```python
from build123d import *

# Parameters (mm, degrees)
PARED_DEPTH           = 25
CONECTORES_REACH      = 165.441
CROQUIS2_W            = 15
CROQUIS2_H            = 13
CROQUIS2_W_2          = 12
CROQUIS2_H_2          = 7
BASE_START            = -1.12
BASE_FRENTE_DEPTH     = 1.12
CORTAR_EXTRUIR2_REACH = 164.686
CROQUIS3_W            = 2
CROQUIS3_H            = 5.5


with BuildPart() as part:
    # Croquis1 → pared (new body)
    with BuildSketch(Plane.XY):
        with BuildLine():
            Line((9, 76.1), (131, 76.1))
            ThreePointArc((131, 76.1), (138.495331881, 72.995331881), (141.6, 65.5))
            Line((141.6, 65.5), (141.6, 9))
            ThreePointArc((141.6, 9), (138.495331881, 1.504668119), (131, -1.6))
            Line((131, -1.6), (9, -1.6))
            ThreePointArc((9, -1.6), (1.504668119, 1.504668119), (-1.6, 9))
            Line((-1.6, 9), (-1.6, 65.5))
            ThreePointArc((-1.6, 65.5), (1.504668119, 72.995331881), (9, 76.1))
        make_face()
        with BuildLine():
            Line((9, 0), (131, 0))
            ThreePointArc((131, 0), (137.363961031, 2.636038969), (140, 9))
            Line((140, 9), (140, 65.5))
            ThreePointArc((140, 65.5), (137.363961031, 71.863961031), (131, 74.5))
            Line((131, 74.5), (9, 74.5))
            ThreePointArc((9, 74.5), (2.636038969, 71.863961031), (0, 65.5))
            Line((0, 65.5), (0, 9))
            ThreePointArc((0, 9), (2.636038969, 2.636038969), (9, 0))
        make_face(mode=Mode.SUBTRACT)
    extrude(amount=PARED_DEPTH)

    # Croquis2 → conectores (cut, up to next)
    with BuildSketch(Plane.XZ.offset(1.6), mode=Mode.PRIVATE) as conectores_sk1:
        with Locations((111, 9.5)):
            Rectangle(CROQUIS2_W, CROQUIS2_H)
    conectores_tool1 = extrude(conectores_sk1.sketch, amount=-CONECTORES_REACH, mode=Mode.PRIVATE) & part.part
    # Croquis2 → conectores (cut, up to next)
    with BuildSketch(Plane.XZ.offset(1.6), mode=Mode.PRIVATE) as conectores_sk2:
        with Locations((96, 14.5)):
            Rectangle(CROQUIS2_W_2, CROQUIS2_H_2)
    conectores_tool2 = extrude(conectores_sk2.sketch, amount=-CONECTORES_REACH, mode=Mode.PRIVATE) & part.part
    add(conectores_tool1.solids().sort_by_distance((111, -1.6, 9.5))[0], mode=Mode.SUBTRACT)
    add(conectores_tool2.solids().sort_by_distance((96, -1.6, 14.5))[0], mode=Mode.SUBTRACT)

    # Croquis1_2 → base frente (add)
    with BuildSketch(Plane.XY.offset(BASE_START)):
        with BuildLine():
            Line((9, 76.1), (131, 76.1))
            ThreePointArc((131, 76.1), (138.495331881, 72.995331881), (141.6, 65.5))
            Line((141.6, 65.5), (141.6, 9))
            ThreePointArc((141.6, 9), (138.495331881, 1.504668119), (131, -1.6))
            Line((131, -1.6), (9, -1.6))
            ThreePointArc((9, -1.6), (1.504668119, 1.504668119), (-1.6, 9))
            Line((-1.6, 9), (-1.6, 65.5))
            ThreePointArc((-1.6, 65.5), (1.504668119, 72.995331881), (9, 76.1))
        make_face()
    extrude(amount=BASE_FRENTE_DEPTH)

    # Croquis3 → Cortar-Extruir2 (cut, up to next)
    with BuildSketch(Plane.XY, mode=Mode.PRIVATE) as cortar_extruir2_sk1:
        with BuildLine():
            Line((131.5, 13), (132.5, 13))
            ThreePointArc((132.5, 13), (132.853553391, 13.146446609), (133, 13.5))
            Line((133, 13.5), (133, 27.5))
            ThreePointArc((133, 27.5), (132.853553391, 27.853553391), (132.5, 28))
            Line((132.5, 28), (131.5, 28))
            ThreePointArc((131.5, 28), (131.146446609, 27.853553391), (131, 27.5))
            Line((131, 27.5), (131, 13.5))
            ThreePointArc((131, 13.5), (131.146446609, 13.146446609), (131.5, 13))
        make_face()
    cortar_extruir2_tool1 = extrude(cortar_extruir2_sk1.sketch, amount=-CORTAR_EXTRUIR2_REACH, mode=Mode.PRIVATE) & part.part
    # Croquis3 → Cortar-Extruir2 (cut, up to next)
    with BuildSketch(Plane.XY, mode=Mode.PRIVATE) as cortar_extruir2_sk2:
        with BuildLine():
            Line((133, 34.5), (131, 34.5))
            Line((131, 34.5), (131, 29.5))
            ThreePointArc((131, 29.5), (131.146446609, 29.146446609), (131.5, 29))
            Line((131.5, 29), (132.5, 29))
            ThreePointArc((132.5, 29), (132.853553391, 29.146446609), (133, 29.5))
            Line((133, 29.5), (133, 34.5))
        make_face()
    cortar_extruir2_tool2 = extrude(cortar_extruir2_sk2.sketch, amount=-CORTAR_EXTRUIR2_REACH, mode=Mode.PRIVATE) & part.part
    # Croquis3 → Cortar-Extruir2 (cut, up to next)
    with BuildSketch(Plane.XY, mode=Mode.PRIVATE) as cortar_extruir2_sk3:
        with Locations((132, 38.25)):
            Rectangle(CROQUIS3_W, CROQUIS3_H)
    cortar_extruir2_tool3 = extrude(cortar_extruir2_sk3.sketch, amount=-CORTAR_EXTRUIR2_REACH, mode=Mode.PRIVATE) & part.part
    # Croquis3 → Cortar-Extruir2 (cut, up to next)
    with BuildSketch(Plane.XY, mode=Mode.PRIVATE) as cortar_extruir2_sk4:
        with Locations((132, 44.75)):
            Rectangle(CROQUIS3_W, CROQUIS3_H)
    cortar_extruir2_tool4 = extrude(cortar_extruir2_sk4.sketch, amount=-CORTAR_EXTRUIR2_REACH, mode=Mode.PRIVATE) & part.part
    # Croquis3 → Cortar-Extruir2 (cut, up to next)
    with BuildSketch(Plane.XY, mode=Mode.PRIVATE) as cortar_extruir2_sk5:
        with BuildLine():
            Line((131, 53.5), (131, 48.5))
            Line((131, 48.5), (133, 48.5))
            Line((133, 48.5), (133, 53.5))
            ThreePointArc((133, 53.5), (132.853553391, 53.853553391), (132.5, 54))
            Line((132.5, 54), (131.5, 54))
            ThreePointArc((131.5, 54), (131.146446609, 53.853553391), (131, 53.5))
        make_face()
    cortar_extruir2_tool5 = extrude(cortar_extruir2_sk5.sketch, amount=-CORTAR_EXTRUIR2_REACH, mode=Mode.PRIVATE) & part.part
    add(cortar_extruir2_tool1.solids().sort_by_distance((132, 20.5, 0))[0], mode=Mode.SUBTRACT)
    add(cortar_extruir2_tool2.solids().sort_by_distance((132, 31.775989, 0))[0], mode=Mode.SUBTRACT)
    add(cortar_extruir2_tool3.solids().sort_by_distance((132, 38.25, 0))[0], mode=Mode.SUBTRACT)
    add(cortar_extruir2_tool4.solids().sort_by_distance((132, 44.75, 0))[0], mode=Mode.SUBTRACT)
    add(cortar_extruir2_tool5.solids().sort_by_distance((132, 51.224011, 0))[0], mode=Mode.SUBTRACT)


solid = part.part
```
The model under review builds one solid part; all positions refer to its coordinate system, in mm. A direction names the side the tool comes from. Coordinates: 2 decimals unless noted, no trailing zeros. Write each loop counter-clockwise with the first axis right and the second up, starting at its lowest first coordinate (ties: lowest second). Pieces come first, ordered by that corner, then holes.
1) We need section D-D on x = 37.5. State the section outline as (y, z) points.
2) We need section B-B on z = 19.75. State the section outline as (x, y) points.
3) Machinability: for faces 5 (the face through (1.59, 1.42, 11.76)), 6 (the face through (71, 38, 0)), which of the approach directions +Z, -Z, +X, -X, +Y, -Y give a long, thin tool a straight path to every point of the face, cutting with its end or side? Answer none if there is none.
4) We need section A-A on x = 91.5. State the section outline as (y, z) points.
5) Clearance check with flat-ended pins moving along their axes: pin 1 Ø3 at (y, z) = (66, 12) entering from -X; pin 2 Ø2 at (x, z) = (116, 9.5) entering from -Y; pin 3 Ø0.5 at (x, z) = (132, -0.5) entering from -Y; pin 4 Ø12 at (x, y) = (92.5, 49) entering from +Z. State where each tip first meets the part, or that it passes through.
6) We need section C-C on y = 57.5. State the section outline as (x, z) points, then the cut area to 3 significant figures.
7) To check wall thickness, follow probe 1 along Y at (x, z) = (117, 1.75); probe 2 along X at (y, z) = (48.5, 22.75); probe 3 along Z at (x, y) = (123.5, 56). State the ranges of each line that lie inside material, in increasing order.
8) The part is to be moulded in two halves that separate along X. For faces 1 (the face through (137.294, 2.566, 12.325)), 2 (the face through (2.566, 2.706, 12.325)), 3 (the face through (70, 75, 25)), 4 (the face through (141.6, 38, 12)), say which applies: pulls with the +X half, pulls with the -X half, needs draft (parallel to the pull), parting line crosses it, or undercut.
Answer list:
1. outline: (-1.6, -1.12) - (76.1, -1.12) - (76.1, 25) - (74.5, 25) - (74.5, 0) - (0, 0) - (0, 25) - (-1.6, 25) - close
2. outline: (-1.6, 9) arc R10.6 ccw to (9, -1.6) - (131, -1.6) arc R10.6 ccw to (141.6, 9) - (141.6, 65.5) arc R10.6 ccw to (131, 76.1) - (9, 76.1) arc R10.6 ccw to (-1.6, 65.5) - close; hole (0, 9) arc R9 ccw to (9, 0) - (131, 0) arc R9 ccw to (140, 9) - (140, 65.5) arc R9 ccw to (131, 74.5) - (9, 74.5) arc R9 ccw to (0, 65.5) - close
3. face 5: +Z, -Z, -X, -Y
3. face 6: +Z
4. outline: (-1.6, -1.12) - (76.1, -1.12) - (76.1, 25) - (74.5, 25) - (74.5, 0) - (0, 0) - (0, 11) - (-1.6, 11) - close; (-1.6, 18) - (0, 18) - (0, 25) - (-1.6, 25) - close
5. pin 1: stops at x = -1.6
5. pin 2: stops at y = 74.5
5. pin 3: stops at y = -1.57
5. pin 4: stops at z = 0
6. outline: (-1.6, -1.12) - (141.6, -1.12) - (141.6, 25) - (140, 25) - (140, 0) - (0, 0) - (0, 25) - (-1.6, 25) - close
6. area: 240 mm2
7. probe 1: y = -1.6 to 0, 74.5 to 76.1
7. probe 2: x = -1.6 to 0, 140 to 141.6
7. probe 3: z = -1.12 to 0
8. face 1: undercut
8. face 2: undercut
8. face 3: needs draft
8. face 4: pulls with the +X half
